from build123d import *

# Parameters (mm, degrees)
F0_R     = 12.75
F0_R_2   = 0.75
F0_R_3   = 4
F0_R_4   = 3
F0_R_5   = 1.5
F1_DEPTH = 2.5
F2_DEPTH = 3


with BuildPart() as f1:
    # F0 (on Top) → F1 (new body)
    with BuildSketch(Plane.XY):
        Circle(F0_R)
        with Locations((-6.3639610307, -6.3639610307)):
            Circle(F0_R_2, mode=Mode.SUBTRACT)
        with Locations((0, -9)):
            Circle(F0_R_2, mode=Mode.SUBTRACT)
        with Locations((6.3639610307, -6.3639610307)):
            Circle(F0_R_2, mode=Mode.SUBTRACT)
        with Locations((-9, 0)):
            Circle(F0_R_2, mode=Mode.SUBTRACT)
        with Locations((-6.3639610307, 6.3639610307)):
            Circle(F0_R_2, mode=Mode.SUBTRACT)
        Circle(F0_R_3, mode=Mode.SUBTRACT)
        with Locations((6.3639610307, 6.3639610307)):
            Circle(F0_R_2, mode=Mode.SUBTRACT)
        with Locations((9, 0)):
            Circle(F0_R_2, mode=Mode.SUBTRACT)
        with Locations((0, 9)):
            Circle(F0_R_2, mode=Mode.SUBTRACT)
        Circle(F0_R_3)
        Circle(F0_R_4, mode=Mode.SUBTRACT)
        Circle(F0_R_4)
        Circle(F0_R_5, mode=Mode.SUBTRACT)
    extrude(amount=F1_DEPTH)

    # F0 (on Top) → F2 (join)
    with BuildSketch(Plane.XY):
        Circle(F0_R_3)
        Circle(F0_R_4, mode=Mode.SUBTRACT)
    extrude(amount=-F2_DEPTH)


solid = f1.part
Geometry check sheet. Reference: the model listing, model coordinates, mm. A direction names the side the tool comes from. Round coordinates to 2 decimals unless told otherwise and drop trailing zeros. Loops run counter-clockwise (first coordinate to the right, second up) from the corner with the lowest first, then second, coordinate; pieces in that order, holes last. Notation, with made-up numbers: (8, 29) -> (47, 29) arc R30 cw to (47, 53) -> close; hole circle Ø5 at (84.25, 34.5). An arc over 180 degrees is marked (long way). Answer as a JSON object with one key per item and string values. Group by question number.
Item 1: Thickness scan on line 1 along Y through (x, z) = (0, 1.1); line 2 along Y through (x, z) = (6.5, 0.1); line 3 along Y through (x, z) = (-1.75, -0.7). Record the ranges inside material, lowest first.
Item 2: Cross-section at A-A, the plane y = 0. Record the cut outline in (x, z).
Item 3: Cross-section at D-D, the plane y = 9. Record the cut outline in (x, z), plus the area to 3 significant figures.
Item 4: Cross-section at C-C, the plane z = 0.5. Count the separate pieces of the cut face and the enclosed holes in it, plus the area to 4 significant figures.
Item 5: Depth check by flat-ended pin: pin 1 Ø3.5 at (x, y) = (0, 0) entering from -Z; pin 2 Ø1 at (x, z) = (3, 0) entering from +Y; pin 3 Ø10 at (x, y) = (7, 4) entering from -Z; pin 4 Ø1 at (y, z) = (-3.5, 1) entering from +X. Enter the tip coordinate at first touch or a pass-through.
Item 6: Set-up check for faces 4 (the face through (5.81, 6.87, 1.23)), 5 (the face through (-0.867, -3.905, -1.479)): record each of +Z, -Z, +X, -X, +Y, -Y from which the full face is reachable in a straight line by a thin tool's end or side.
Item 7: Release check for a two-part mould opening along Y. For faces 1 (the face through (-0.098, 9.744, 1.232)), 2 (the face through (-2.764, -12.447, 1.232)), 3 (the face through (3, 0, 2.5)) record: pulls with the +Y half, pulls with the -Y half, needs draft (parallel to the pull), parting line crosses it, or undercut.
Determined:
{
 "1": {"line 1": "y = -12.75 to -9.75, -8.25 to -1.5, 1.5 to 8.25, 9.75 to 12.75", "line 2": "y = -10.97 to -7.1, -5.63 to 5.63, 7.1 to 10.97", "line 3": "y = -3.6 to -2.44, 2.44 to 3.6"},
 "2": {"outline": "(-12.75, 0) -> (-9.75, 0) -> (-9.75, 2.5) -> (-12.75, 2.5) -> close; (-8.25, 0) -> (-4, 0) -> (-4, -3) -> (-3, -3) -> (-3, 0) -> (-1.5, 0) -> (-1.5, 2.5) -> (-8.25, 2.5) -> close; (1.5, 0) -> (3, 0) -> (3, -3) -> (4, -3) -> (4, 0) -> (8.25, 0) -> (8.25, 2.5) -> (1.5, 2.5) -> close; (9.75, 0) -> (12.75, 0) -> (12.75, 2.5) -> (9.75, 2.5) -> close"},
 "3": {"outline": "(-9.03, 0) -> (-0.75, 0) -> (-0.75, 2.5) -> (-9.03, 2.5) -> close; (0.75, 0) -> (9.03, 0) -> (9.03, 2.5) -> (0.75, 2.5) -> close", "area": "41.4 mm²"},
 "4": {"separate pieces": "1", "enclosed holes": "9", "area": "489.5 mm²"},
 "5": {"pin 1": "stops at z = 0", "pin 2": "stops at y = 12.5", "pin 3": "stops at z = -3", "pin 4": "stops at x = 12.39"},
 "6": {"face 4": "+Z, -Z", "face 5": "-Z"},
 "7": {"face 1": "undercut", "face 2": "parting line crosses it", "face 3": "needs draft"}
}
